Answer from the drawing. Dimensions are ordinates in mm from the lowest x, y and z of the part. Give positions to 0.01 mm unless a question says otherwise; leave off trailing zeros. Write each loop counter-clockwise with the first axis right and the second up, starting at its lowest first coordinate (ties: lowest second). Pieces come first, ordered by that corner, then holes. Notation, with made-up numbers: M -26,-3.5 L 4,-3.5 A21 ccw 4,16.5 Z; hole C -17,37 d10. An arc over 180 degrees is marked long. Put each result on its own line as item: value.
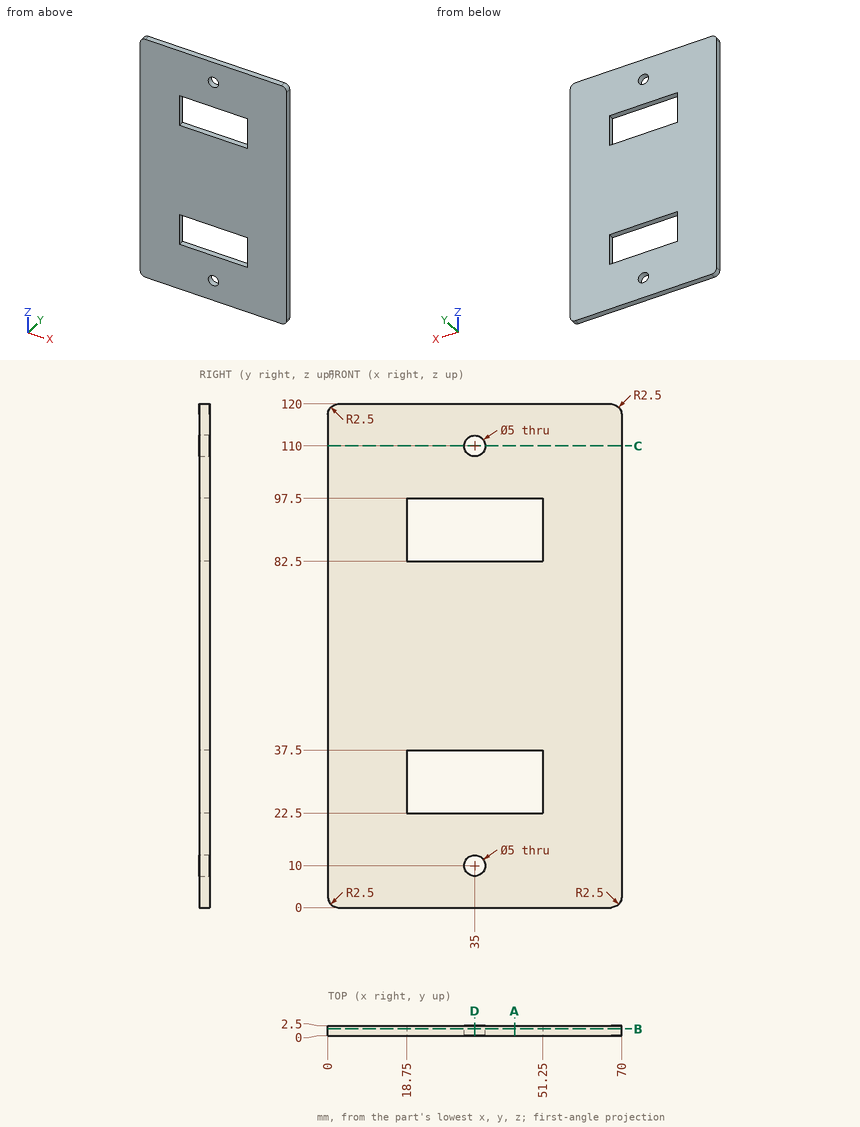
(1) Section C-C on z = 110 is taken. Determine the outline of the cut face in (x, y).
Result:
outline: M 0,0 L 32.5,0 L 32.5,2.5 L 0,2.5 Z; M 37.5,0 L 70,0 L 70,2.5 L 37.5,2.5 Z
(2) Section A-A on x = 44.5 is taken. Determine the outline of the cut face in (y, z), and give its area (3 significant figures).
Result:
outline: M 0,0 L 2.5,0 L 2.5,22.5 L 0,22.5 Z; M 0,37.5 L 2.5,37.5 L 2.5,82.5 L 0,82.5 Z; M 0,97.5 L 2.5,97.5 L 2.5,120 L 0,120 Z
area: 225 mm²
(3) Straight lines are drawn through the part: line 1 along Z through (x, y) = (40.5, 0.35); line 2 along X through (y, z) = (0.75, 10); line 3 along X through (y, z) = (0.2, 26). For each, find the intervals that lie inside material, in ascending order. Write a range as from..to.
Result:
line 1: z = 0..22.5, 37.5..82.5, 97.5..120
line 2: x = 0..32.5, 37.5..70
line 3: x = 0..18.75, 51.25..70
(4) Section B-B on y = 1.7 is taken. Determine the outline of the cut face in (x, z), and give its area (3 significant figures).
Result:
outline: M 0,2.5 A2.5 ccw 2.5,0 L 67.5,0 A2.5 ccw 70,2.5 L 70,117.5 A2.5 ccw 67.5,120 L 2.5,120 A2.5 ccw 0,117.5 Z; hole M 18.75,22.5 L 51.25,22.5 L 51.25,37.5 L 18.75,37.5 Z; hole M 18.75,82.5 L 51.25,82.5 L 51.25,97.5 L 18.75,97.5 Z; hole C 35,10 d5; hole C 35,110 d5
area: 7,380 mm²
(5) Section D-D on x = 35 is taken. Determine the outline of the cut face in (y, z), and give its area (3 significant figures).
Result:
outline: M 0,0 L 2.5,0 L 2.5,7.5 L 0,7.5 Z; M 0,12.5 L 2.5,12.5 L 2.5,22.5 L 0,22.5 Z; M 0,37.5 L 2.5,37.5 L 2.5,82.5 L 0,82.5 Z; M 0,97.5 L 2.5,97.5 L 2.5,107.5 L 0,107.5 Z; M 0,112.5 L 2.5,112.5 L 2.5,120 L 0,120 Z
area: 200 mm²
